Verification items for the finished model (mm, model axes). Face numbers are marked on the shaded views. Coordinates: 2 decimals unless noted, no trailing zeros. Order: outer loops, then holes, each group sorted by start corner. A loop starts at its lowest first (then second) coordinate and runs counter-clockwise, first axis right, second up. Notation, with made-up numbers: M -29,45 L 12,45 A34 cw 12,75 Z; hole C -32.5,83 d1. An arc over 180 degrees is marked long. Use one line per item in the form item = value. Start each with the question number.
```python
from build123d import *

# Parameters (mm, degrees)
SKETCH2_R           = 20
SKETCH2_R_2         = 10
EXTRUDE1_DEPTH      = 420.09
SKETCH3_R           = 20
SKETCH3_R_2         = 15
EXTRUDE2_DEPTH      = 60
EXTRUDE2_DEPTH_BACK = 60
SKETCH4_R           = 20
EXTRUDE3_DEPTH      = 10
SKETCH5_R           = 20
EXTRUDE4_DEPTH      = 10
SKETCH6_R           = 5
EXTRUDE5_DEPTH      = 33
SKETCH7_R           = 5
EXTRUDE6_DEPTH      = 33
SKETCH8_W           = 40
SKETCH8_H           = 40
EXTRUDE7_DEPTH      = 10
SKETCH9_W           = 40
SKETCH9_H           = 5
EXTRUDE8_DEPTH      = 40
SKETCH10_R          = 10
CUT_EXTRUDE1_DEPTH  = 124
FILLET1_R           = 3
FILLET2_R           = 3
SKETCH11_W          = 60
SKETCH11_H          = 100
EXTRUDE9_DEPTH      = 20
FILLET3_R           = 10
FILLET4_R           = 5


with BuildPart() as part:
    # Sketch2 → Extrude1 (new body)
    with BuildSketch(Plane(origin=(0, 0, 0), x_dir=(1, 0, 0), z_dir=(0, 1, 0))):
        with Locations(Location((0, 0, 0), (0, 0, 270))):  # turned: the seam where the file's is
            Circle(SKETCH2_R)
        with Locations(Location((0, 0, 0), (0, 0, 270))):  # turned: the seam where the file's is
            Circle(SKETCH2_R_2, mode=Mode.SUBTRACT)
    extrude(amount=EXTRUDE1_DEPTH)

    # Sketch3 → Extrude2 (add, two sides)
    with BuildSketch(Plane.XY) as extrude2_sk:
        with Locations((0, 20)):
            Circle(SKETCH3_R)
        with Locations(Location((0, 20, 0), (0, 0, 180))):  # turned: the seam where the file's is
            Circle(SKETCH3_R_2, mode=Mode.SUBTRACT)
    extrude(amount=EXTRUDE2_DEPTH)
    extrude(extrude2_sk.sketch, amount=-EXTRUDE2_DEPTH_BACK)

    # Sketch4 → Extrude3 (add)
    with BuildSketch(Plane.XY.offset(60)):
        with Locations((0, 20)):
            Circle(SKETCH4_R)
    extrude(amount=EXTRUDE3_DEPTH)

    # Sketch5 → Extrude4 (add)
    with BuildSketch(Plane(origin=(0, 0, -60), x_dir=(-1, 0, 0), z_dir=(0, 0, -1))):
        with Locations(Location((0, 20, 0), (0, 0, 180))):  # turned: the seam where the file's is
            Circle(SKETCH5_R)
    extrude(amount=EXTRUDE4_DEPTH)

    # Sketch6 → Extrude5 (add)
    with BuildSketch(Plane(origin=(0, 0, -70), x_dir=(-1, 0, 0), z_dir=(0, 0, -1))):
        with Locations((0, 20)):
            Circle(SKETCH6_R)
    extrude(amount=EXTRUDE5_DEPTH)

    # Sketch7 → Extrude6 (add)
    with BuildSketch(Plane.XY.offset(70)):
        with Locations(Location((0, 20, 0), (0, 0, 180))):  # turned: the seam where the file's is
            Circle(SKETCH7_R)
    extrude(amount=EXTRUDE6_DEPTH)

    # Sketch8 → Extrude7 (add)
    with BuildSketch(Plane(origin=(0, 420.09, 0), x_dir=(-1, 0, 0), z_dir=(0, 1, 0))):
        Rectangle(SKETCH8_W, SKETCH8_H)
    extrude(amount=EXTRUDE7_DEPTH)

    # Sketch9 → Extrude8 (add)
    with BuildSketch(Plane(origin=(0, 430.09, 0), x_dir=(-1, 0, 0), z_dir=(0, 1, 0))):
        with Locations((0, 17.5)):
            Rectangle(SKETCH9_W, SKETCH9_H)
        with Locations((0, -17.5)):
            Rectangle(SKETCH9_W, SKETCH9_H)
    extrude(amount=EXTRUDE8_DEPTH)

    # Sketch10 → Cut-Extrude1 (cut, through all)
    with BuildSketch(Plane(origin=(0, 0, -20), x_dir=(-1, 0, 0), z_dir=(0, 0, -1))):
        with Locations((0, 450.09)):
            Circle(SKETCH10_R)
    extrude(amount=-CUT_EXTRUDE1_DEPTH, mode=Mode.SUBTRACT)

    # Fillet1
    fillet1_edges = [part.edges().sort_by_distance(p)[0] for p in [
        (-20, 20, 70),
    ]]
    fillet(fillet1_edges, radius=FILLET1_R)

    # Fillet2
    fillet2_edges = [part.edges().sort_by_distance(p)[0] for p in [
        (-20, 20, -70),
    ]]
    fillet(fillet2_edges, radius=FILLET2_R)

    # Sketch11 → Extrude9 (add)
    with BuildSketch(Plane.XZ.offset(-40)):
        with Locations((-10, 0)):
            Rectangle(SKETCH11_W, SKETCH11_H)
    extrude(amount=EXTRUDE9_DEPTH)

    # Fillet3
    fillet3_edges = [part.edges().sort_by_distance(p)[0] for p in [
        (5, 20, -70),
        (5, 20, 70),
    ]]
    fillet(fillet3_edges, radius=FILLET3_R)

    # Fillet4
    fillet4_edges = [part.edges().sort_by_distance(p)[0] for p in [
        (0, 430.09, -15),
        (0, 430.09, 15),
    ]]
    fillet(fillet4_edges, radius=FILLET4_R)


solid = part.part
```
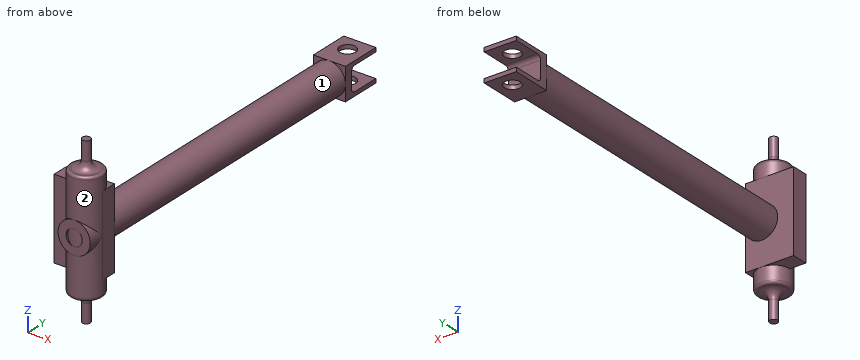
1. Cross-section at B-B on z = -43.5. Enter the section's corners in (x, y), and give its area (3 significant figures).
2. Cross-section at A-A on y = 450.09. Enter the section's corners in (x, z).
3. Cross-section at C-C on z = -88. Enter the section's corners in (x, y).
4. Depth check by flat-ended pin: P1, Ø4, axis at x = -15, y = 51.5, coming from the +Z side; P2, Ø22, axis at x = 11, y = 26, coming from the -Z side; P3, Ø1.5, axis at x = 11.5, y = 165.5, coming from the +Z side; P4, Ø18, axis at x = 0, z = 0, coming from the +Y side. Enter the tip coordinate at first touch or a pass-through.
5. Material ranges on line 1 along X through (y, z) = (17, 0); line 2 along Z through (x, y) = (0, 13.75); line 3 along Z through (x, y) = (-0.5, 344), recorded low to high.
6. Release check for a two-part mould opening along Y. For the marked faces 1 and 2 record: pulls with the +Y half, pulls with the -Y half, needs draft (parallel to the pull), parting line crosses it, or undercut.
Final values:
q1.outline = M -40,20 L -20,20 A20 ccw 20,20 L 20,40 L -40,40 Z; hole M -15,20 A15 ccw 15,20 Z
q1.area = 1,470 mm2
q2.outline = M -20,-20 L -10,-20 L -10,-15 L -20,-15 Z; M -20,15 L -10,15 L -10,20 L -20,20 Z; M 10,-20 L 20,-20 L 20,-15 L 10,-15 Z; M 10,15 L 20,15 L 20,20 L 10,20 Z
q3.outline = C 0,20 d10
q4.P1 = 15.2
q4.P2 = -103
q4.P3 = 16.87
q4.P4 = 430.09
q5.line_1 = -20 to -10, 10 to 20
q5.line_2 = -75.16 to -60, -20 to -10, 10 to 20, 60 to 75.16
q5.line_3 = -19.99 to -9.99, 9.99 to 19.99
q6.face_1 = undercut
q6.face_2 = parting line crosses it
